Verification items for the finished model (mm, model axes). Round coordinates to 2 decimals unless told otherwise and drop trailing zeros. Loops run counter-clockwise (first coordinate to the right, second up) from the corner with the lowest first, then second, coordinate; pieces in that order, holes last. Notation, with made-up numbers: M 44.25,11.25 L 58.25,11.25 A37 ccw 58.25,48.25 Z; hole C -1.5,22.25 d11. An arc over 180 degrees is marked long. One line per item, written item: value.
from build123d import *

# Parameters (mm, degrees)
BOSS_EXTRUDE1_DEPTH = 0.2
FILLET4_R           = 0.1
FILLET5_R           = 0.1


with BuildPart() as part:
    # Sketch2 → Boss-Extrude1 (new body)
    with BuildSketch(Plane(origin=(0, 0, 0), x_dir=(1, 0, 0), z_dir=(0, 1, 0))):
        Polygon((-3, 0), (1e-09, 7.5), (31.5, 0.5), (31.5, -0.5), (1e-09, -7.5), align=None)
    extrude(amount=BOSS_EXTRUDE1_DEPTH)

    # Fillet4
    fillet4_edges = [part.edges().sort_by_distance(p)[0] for p in [
        (31.5, 0.1, 0.5),
    ]]
    fillet(fillet4_edges, radius=FILLET4_R)

    # Fillet5
    fillet5_edges = [part.edges().sort_by_distance(p)[0] for p in [
        (31.5, 0.1, -0.5),
    ]]
    fillet(fillet5_edges, radius=FILLET5_R)


solid = part.part
(1) Sectioned sample at B-B on z = -1.5. Enter the section's corners in (x, y), and give its area (3 significant figures).
Completed:
outline: M -2.4,0 L 27,0 L 27,0.2 L -2.4,0.2 Z
area: 5.88 mm^2
(2) Thickness scan on L1, parallel to Z at x = 25, y = 0.1; L2, parallel to Z at x = 2, y = 0.1. Record the ranges inside material, lowest first. Write a range as from..to.
Completed:
L1: z = -1.94..1.94
L2: z = -7.06..7.06
(3) Sectioned sample at A-A on y = 0.15. Enter the section's corners in (x, z), and give its area (3 significant figures).
Completed:
outline: M -3,0 L 0,-7.5 L 31.42,-0.52 A0.1 ccw 31.5,-0.42 L 31.5,0.42 A0.1 ccw 31.42,0.52 L 0,7.5 Z
area: 274 mm^2
(4) Sectioned sample at C-C on x = 26.5. Enter the section's corners in (y, z).
Completed:
outline: M 0,-1.61 L 0.2,-1.61 L 0.2,1.61 L 0,1.61 Z
